The model under review builds one solid part; all positions refer to its coordinate system, in mm. A direction names the side the tool comes from. Give positions to 0.01 mm unless a question says otherwise; leave off trailing zeros. Order: outer loops, then holes, each group sorted by start corner. A loop starts at its lowest first (then second) coordinate and runs counter-clockwise, first axis right, second up. Notation, with made-up numbers: M -14.5,56.25 L 22.5,56.25 A24 ccw 22.5,94.25 Z; hole C 63,61 d7. An arc over 180 degrees is marked long. One line per question, with ' | ' between items. Start each with the question number.
1. We need section A-A on z = 22. Write out the cut boundary in (x, y).
2. We need section B-B on y = 7.5. Write out the cut boundary in (x, z).
3. We need section C-C on x = 16.5. Write out the cut boundary in (y, z) (1 decimal).
4. Insertion check: P1, Ø7.5, axis at x = 74.93, y = 40.81, coming from the +Z side; P2, Ø10, axis at x = 62, y = 31.5, coming from the -Z side; P3, Ø5, axis at x = -3, y = 42.5, coming from the -Z side; P4, Ø10, axis at y = 35.5, z = 29, coming from the -X side. Each pin has a flat end and moves straight along its axis. Give the tip position at first contact, or say it passes through.
5. For faces 4 (the face through (-3, 25.229, 44)), 5 (the face through (181, 38, 6.35)), 6 (the face through (181, 50.943, 44)), 7 (the face through (-25.13, 37.79, 79.53)), 8 (the face through (36.517, 41.022, 5.149)), list the 3-axis set-ups (+Z, -Z, +X, -X, +Y, -Y) from which the entire face can be reached by the end or side of a thin tool; tool diameter is ignored.
6. We need section D-D on z = 63. Write out the cut boundary in (x, y), then the cut area to 3 significant figures.
7. Wall thickness on L1, parallel to X at y = 33.5, z = 14; L2, parallel to Z at x = 67, y = 55.5; L3, parallel to X at y = 56.5, z = 17: over which ranges is each line inside the solid? List them lowest first.
8. The part is to be moulded in two halves that separate along Y. For faces 1 (the face through (131.767, 41.022, 5.149)), 2 (the face through (209.194, 36.654, 73.012)), 3 (the face through (-3, 38, 82.434)), say which applies: +Y half, -Y half, draft (parallel to the pull), parting line (faces both ways), or undercut.
```python
from build123d import *

# Parameters (mm, degrees)
F0_W      = 177.8
F0_H      = 38.1
F1_DEPTH  = 76.2
F3_DEPTH  = 6.35
F5_DEPTH  = 6.35
F7_DEPTH  = 76.2
F8_R      = 3.4925
F9_DEPTH  = 228.6
F10_R     = 4.7625
F11_DEPTH = 38.1
F12_R     = 3.443795
F13_DEPTH = 279.4


with BuildPart() as f1:
    # F0 (on Front) → F1 (new body)
    with BuildSketch(Plane.XZ):
        with Locations((88.9, 19.05)):
            Rectangle(F0_W, F0_H)
    extrude(amount=-F1_DEPTH)

    # F2 (on face) → F3 (join)
    with BuildSketch(Plane.YZ.offset(177.8)):
        Polygon((25.543192, 82.55), (25.543192, 6.35), (38.1, 6.35), (50.943192, 6.35), (50.943192, 82.55), align=None)
    extrude(amount=F3_DEPTH)

    # F4 (on face) → F5 (join)
    with BuildSketch(Plane(origin=(0, 0, 0), x_dir=(0, -1, 0), z_dir=(-1, 0, 0))):
        Polygon((-50.629251, 82.433985), (-50.629251, 6.233985), (-38.072443, 6.233985), (-25.229251, 6.233985), (-25.229251, 82.433985), align=None)
    extrude(amount=F5_DEPTH)

    # F6 (on face) → F7 (cut)
    with BuildSketch(Plane.XZ):
        Polygon((25.4, 29.206271), (25.4, 19.681271), (25.4, 10.156271), (152.4, 10.156271), (152.4, 19.681271), (152.4, 29.206271), align=None)
    extrude(amount=-F7_DEPTH, mode=Mode.SUBTRACT)

    # F8 (on face) → F9 (join)
    with BuildSketch(Plane.YZ.offset(184.15)):
        with Locations((38.243192, 76.067708)):
            Circle(F8_R)
    extrude(amount=-F9_DEPTH)

    # F10 (on face) → F11 (cut)
    with BuildSketch(Plane.XY.offset(38.1)):
        with BuildLine():
            ThreePointArc((43.284044, 59.817001), (41.275, 60.261499), (39.265956, 59.817001))
            Line((39.265956, 59.817001), (43.284044, 59.817001))
        make_face()
        with BuildLine():
            ThreePointArc((138.534044, 59.817001), (136.525, 60.261499), (134.515956, 59.817001))
            Line((134.515956, 59.817001), (138.534044, 59.817001))
        make_face()
        with BuildLine():
            Line((138.534044, 59.817001), (134.515956, 59.817001))
            ThreePointArc((134.515956, 59.817001), (133.964401, 51.483436), (141.2875, 55.498999))
            ThreePointArc((141.2875, 55.498999), (140.540562, 58.059597), (138.534044, 59.817001))
        make_face()
        with BuildLine():
            ThreePointArc((106.784044, 59.817001), (104.775, 60.261499), (102.765956, 59.817001))
            Line((102.765956, 59.817001), (106.784044, 59.817001))
        make_face()
        with BuildLine():
            Line((106.784044, 59.817001), (102.765956, 59.817001))
            ThreePointArc((102.765956, 59.817001), (102.214401, 51.483436), (109.5375, 55.498999))
            ThreePointArc((109.5375, 55.498999), (108.790562, 58.059597), (106.784044, 59.817001))
        make_face()
        with BuildLine():
            ThreePointArc((76.939042, 59.817001), (74.929997, 60.261499), (72.920953, 59.817001))
            Line((72.920953, 59.817001), (76.939042, 59.817001))
        make_face()
        with BuildLine():
            Line((76.939042, 59.817001), (72.920953, 59.817001))
            ThreePointArc((72.920953, 59.817001), (72.369399, 51.483436), (79.692497, 55.498999))
            ThreePointArc((79.692497, 55.498999), (78.94556, 58.059597), (76.939042, 59.817001))
        make_face()
        with BuildLine():
            Line((43.284044, 59.817001), (39.265956, 59.817001))
            ThreePointArc((39.265956, 59.817001), (38.714401, 51.483436), (46.0375, 55.498999))
            ThreePointArc((46.0375, 55.498999), (45.290562, 58.059597), (43.284044, 59.817001))
        make_face()
        with Locations((41.275, 40.812645)):
            Circle(F10_R)
        with Locations((74.929997, 40.812645)):
            Circle(F10_R)
        with Locations((104.775, 40.812645)):
            Circle(F10_R)
        with Locations((136.525, 40.812645)):
            Circle(F10_R)
        with Locations((41.275, 25.229251)):
            Circle(F10_R)
        with Locations((74.929997, 25.229251)):
            Circle(F10_R)
        with Locations((104.775, 25.229251)):
            Circle(F10_R)
        with Locations((136.525, 25.229251)):
            Circle(F10_R)
    extrude(amount=-F11_DEPTH, mode=Mode.SUBTRACT)

    # F12 (on face) → F13 (join)
    with BuildSketch(Plane(origin=(-44.45, 0, 0), x_dir=(0, -1, 0), z_dir=(-1, 0, 0))):
        with Locations((-38.243192, 76.067708)):
            Circle(F12_R)
    extrude(amount=-F13_DEPTH)


solid = f1.part
```
Entries:
1) outline: M -6.35,25.23 L 0,25.23 L 0,0 L 25.4,0 L 25.4,76.2 L 0,76.2 L 0,50.63 L -6.35,50.63 Z; M 152.4,0 L 177.8,0 L 177.8,25.54 L 184.15,25.54 L 184.15,50.94 L 177.8,50.94 L 177.8,76.2 L 152.4,76.2 Z
2) outline: M 0,0 L 177.8,0 L 177.8,38.1 L 0,38.1 Z; hole M 25.4,10.16 L 152.4,10.16 L 152.4,29.21 L 25.4,29.21 Z
3) outline: M 0,0 L 76.2,0 L 76.2,38.1 L 0,38.1 Z; C 38.2,76.1 d7
4) P1: stops at z = 79.56 | P2: stops at z = 0 | P3: stops at z = 6.23 | P4: stops at x = -6.35
5) face 4: +Z, -Z, -X, -Y | face 5: -Z, +X, +Y, -Y | face 6: +Z, -Z, +X, +Y | face 7: -X | face 8: -Z
6) outline: M -6.35,25.23 L 0,25.23 L 0,50.63 L -6.35,50.63 Z; M 177.8,25.54 L 184.15,25.54 L 184.15,50.94 L 177.8,50.94 Z | area: 323 mm^2
7) L1: x = -6.35 to 25.4, 152.4 to 184.15 | L2: z = 0 to 10.16, 29.21 to 38.1 | L3: x = 0 to 25.4, 152.4 to 177.8
8) face 1: undercut | face 2: parting line | face 3: draft
